```python
from build123d import *

# Parameters (mm, degrees)
SALIENTE_EXTRUIR1_DEPTH = 8
REDONDEO1_R             = 3


with BuildPart() as part:
    # Croquis1 → Saliente-Extruir1 (new body)
    with BuildSketch(Plane.XY):
        Polygon((-13.6, 3.644109017), (0, 0), (0, 13.644109017), (-13.6, 13.644109017), align=None)
    extrude(amount=SALIENTE_EXTRUIR1_DEPTH)

    # Redondeo1
    redondeo1_edges = [part.edges().sort_by_distance(p)[0] for p in [
        (0, 13.644109017, 4),
        (-13.6, 13.644109017, 4),
    ]]
    fillet(redondeo1_edges, radius=REDONDEO1_R)


solid = part.part
```
Read the model definition and answer for the solid it produces. Units are mm, in the model's axes. Coordinates: 2 decimals unless noted, no trailing zeros. Loops run counter-clockwise (first coordinate to the right, second up) from the corner with the lowest first, then second, coordinate; pieces in that order, holes last. Notation, with made-up numbers: (82.25, 25.25) -> (113.25, 25.25) arc R27 cw to (113.25, 61.25) -> close; hole circle Ø9 at (68.25, -25.5). An arc over 180 degrees is marked (long way). Return JSON: item names as keys, results as strings.
Item 1: A flat-ended cylindrical pin translates along its axis: P1, Ø2, axis at x = -4.5, z = 2, coming from the -Y side. Find the tip coordinate at first contact, or state that the pin passes through.
Answers:
{"P1": "stops at y = 0.94"}
Item 2: Find section B-B (x = -2.25). Determine the outline of the cut face in (y, z), plus the area to 3 significant figures.
Answers:
{"outline": "(0.6, 0) -> (13.55, 0) -> (13.55, 8) -> (0.6, 8) -> close", "area": "104 mm2"}
Item 3: Find section A-A (z = 4.5). Determine the outline of the cut face in (x, y).
Answers:
{"outline": "(-13.6, 3.64) -> (0, 0) -> (0, 10.64) arc R3 ccw to (-3, 13.64) -> (-10.6, 13.64) arc R3 ccw to (-13.6, 10.64) -> close"}
Item 4: Find section C-C (y = 2.75). Determine the outline of the cut face in (x, z), plus the area to 3 significant figures.
Answers:
{"outline": "(-10.26, 0) -> (0, 0) -> (0, 8) -> (-10.26, 8) -> close", "area": "82.1 mm2"}
Item 5: Find the intervals of material crossed by probe 1 along Y at (x, z) = (-9.5, 5); probe 2 along Y at (x, z) = (-8.5, 0.75); probe 3 along X at (y, z) = (11.75, 4), in increasing order.
Answers:
{"probe 1": "y = 2.55 to 13.64", "probe 2": "y = 2.28 to 13.64", "probe 3": "x = -13.39 to -0.21"}
Item 6: For a pull along X with two mould halves and no side action, classify faces 1 (the flat face through (-7, 7, 0)), 2 (the flat face through (-13.6, 7, 4)), 3 (the flat face through (0, 5, 4)) as +X half, -X half, draft (parallel to the pull), parting line (faces both ways), or undercut.
Answers:
{"face 1": "draft", "face 2": "-X half", "face 3": "+X half"}
